Build history of the part. All positions in model axes, mm. A direction names the side the tool comes from. Give positions to 0.01 mm unless a question says otherwise; leave off trailing zeros. Order: outer loops, then holes, each group sorted by start corner. A loop starts at its lowest first (then second) coordinate and runs counter-clockwise, first axis right, second up. Notation, with made-up numbers: (56, 8.25) -> (60, 8.25) arc R8 cw to (60, 16.25) -> close; hole circle Ø10 at (58.25, 13). An arc over 180 degrees is marked (long way). One line per item, written item: value. Start each with the question number.
(1) Probe line 1 (Y direction, x = 0, z = 53.9); line 2 (Z direction, x = -0.75, y = -2); line 3 (Y direction, x = -1.25, z = 33). List the from-to ranges inside material, lowest first.
(2) Pin check, flat tips, straight feed: pin 1 (1.5 mm diameter, centred on y = -17, z = 43, fed in from +X); pin 2 (4.5 mm diameter, centred on x = 2.5, y = 1, fed in from -Z); pin 3 (4 mm diameter, centred on y = -3.5, z = 47, fed in from -X); pin 4 (2.5 mm diameter, centred on x = 0, z = 25.5, fed in from +Y). Stop position of each tip, or through.
(3) Which spindle directions (+Z, -Z, +X, -X, +Y, -Y) get a long thin tool onto all of the face, cutting with end or side? Do faces 4 (the cylindrical face through (-1.5, 0.07, 53.54)), 5 (the flat face through (-2.318, -12, 28)), 6 (the flat face through (2, -5.743, 28)). Say none if no direction does.
(4) Saw through at D-D on y = -9.5. Give the cut face in (x, z).
(5) Saw through at C-C on x = 5. Give the cut face in (y, z).
(6) Two-plate mould, pull along Y, no slides. Class faces 1 (the flat face through (-2.163, 1.372, 2.465)), 2 (the cylindrical face through (3.22, 0.09, 2.46)), 3 (the cylindrical face through (-4.35, -1.62, 53.54)): +Y half, -Y half, draft (parallel to the pull), parting line (faces both ways), or undercut.
(7) Saw through at A-A on x = 0. Give the cut face in (y, z).
(8) Saw through at B-B on z = 14.5. Give the cut face in (x, y), plus the area to 3 significant figures.
```python
from build123d import *

# Parameters (mm, degrees)
SKETCH1_R           = 1.5
BOSS_EXTRUDE1_DEPTH = 5
BOSS_EXTRUDE2_DEPTH = 23


with BuildPart() as part:
    # Sketch1 → Boss-Extrude1 (new body)
    with BuildSketch(Plane.XY):
        with BuildLine():
            Line((-3.762452186, -3.055345405), (-3.196477247, -3.621320344))
            ThreePointArc((-3.196477247, -3.621320344), (-2.546158993, -4.59459039), (-2.31779759, -5.742640687))
            Line((-2.31779759, -5.742640687), (-2.31779759, -18.5))
            ThreePointArc((-2.31779759, -18.5), (-2.024904371, -19.207106781), (-1.31779759, -19.5))
            Line((-1.31779759, -19.5), (18.54616344, -19.5))
            ThreePointArc((18.54616344, -19.5), (19.008103207, -19.191341716), (18.899716831, -18.646446609))
            Line((18.899716831, -18.646446609), (2.601508845, -2.348238623))
            ThreePointArc((2.601508845, -2.348238623), (2.308615626, -1.641131842), (2.601508845, -0.934025061))
            Line((2.601508845, -0.934025061), (2.927422074, -0.608111832))
            ThreePointArc((2.927422074, -0.608111832), (3.220315293, 0.098994949), (2.927422074, 0.806101731))
            Line((2.927422074, 0.806101731), (0.806101731, 2.927422074))
            ThreePointArc((0.806101731, 2.927422074), (0.098994949, 3.220315293), (-0.608111832, 2.927422074))
            Line((-0.608111832, 2.927422074), (-1.641131842, 1.894402064))
            Line((-1.641131842, 1.894402064), (-3.762452186, -0.22691828))
            ThreePointArc((-3.762452186, -0.22691828), (-4.348238623, -1.641131842), (-3.762452186, -3.055345405))
        make_face()
        Circle(SKETCH1_R, mode=Mode.SUBTRACT)
    boss_extrude1 = extrude(amount=BOSS_EXTRUDE1_DEPTH)

    # Sketch2 → Boss-Extrude2 (add)
    with BuildSketch(Plane.XY.offset(5)):
        with BuildLine():
            Line((18.899716831, -18.646446609), (5.995910909, -5.742640687))
            Line((5.995910909, -5.742640687), (-2.31779759, -5.742640687))
            Line((-2.31779759, -5.742640687), (-2.31779759, -18.5))
            ThreePointArc((-2.31779759, -18.5), (-2.024904371, -19.207106781), (-1.31779759, -19.5))
            Line((-1.31779759, -19.5), (18.54616344, -19.5))
            ThreePointArc((18.54616344, -19.5), (19.008103207, -19.191341716), (18.899716831, -18.646446609))
        make_face()
    boss_extrude2 = extrude(amount=BOSS_EXTRUDE2_DEPTH)

    # Mirror1: Boss-Extrude1, Boss-Extrude2 across plane
    add(boss_extrude1.mirror(Plane.XY.offset(28)))
    add(boss_extrude2.mirror(Plane.XY.offset(28)))


solid = part.part
```
Results below:
1. line 1: y = -19.5 to -1.5, 1.5 to 3.22
1. line 2: z = 0 to 5, 51 to 56
1. line 3: y = -19.5 to -5.74
2. pin 1: stops at x = 18
2. pin 2: stops at z = 0
2. pin 3: passes through
2. pin 4: stops at y = -5.74
3. face 4: +Z, -Z
3. face 5: +Z, -Z, -X, -Y
3. face 6: +X, -X, +Y
4. outline: (-2.32, 0) -> (9.75, 0) -> (9.75, 56) -> (-2.32, 56) -> close
5. outline: (-19.5, 0) -> (-4.75, 0) -> (-4.75, 5) -> (-5.74, 5) -> (-5.74, 51) -> (-4.75, 51) -> (-4.75, 56) -> (-19.5, 56) -> close
6. face 1: +Y half
6. face 2: undercut
6. face 3: parting line
7. outline: (-19.5, 0) -> (-1.5, 0) -> (-1.5, 5) -> (-5.74, 5) -> (-5.74, 51) -> (-1.5, 51) -> (-1.5, 56) -> (-19.5, 56) -> close; (1.5, 0) -> (3.22, 0) -> (3.22, 5) -> (1.5, 5) -> close; (1.5, 51) -> (3.22, 51) -> (3.22, 56) -> (1.5, 56) -> close
8. outline: (-2.32, -18.5) arc R1 ccw to (-1.32, -19.5) -> (18.55, -19.5) arc R0.5 ccw to (18.9, -18.65) -> (6, -5.74) -> (-2.32, -5.74) -> close
8. area: 208 mm²
